For this review, take the finished solid that the model builds, in its own axes (mm). Face numbers are marked on the shaded views. A direction names the side the tool comes from. Coordinates: 2 decimals unless noted, no trailing zeros. Order: outer loops, then holes, each group sorted by start corner. A loop starts at its lowest first (then second) coordinate and runs counter-clockwise, first axis right, second up. Notation, with made-up numbers: M -8,-35 L 42,-35 A13 ccw 42,-20 Z; hole C 22.5,-36 d3. An arc over 180 degrees is marked long. Use CSV: the item, a comma, the result in double quotes.
```python
from build123d import *

# Parameters (mm, degrees)
F1_DEPTH = 50.8
F2_R     = 5.08
F3_R     = 5.08
F4_R     = 3.175
F5_DEPTH = 25.4


with BuildPart() as f1:
    # F0 (on Front) → F1 (new body)
    with BuildSketch(Plane.XZ):
        with BuildLine():
            Line((-25, -25), (-25, 0))
            Line((-25, 0), (-20, 0))
            ThreePointArc((-20, 0), (0, 20), (20, 0))
            Line((20, 0), (25, 0))
            Line((25, 0), (25, -25))
            Line((25, -25), (46.55, -25))
            Line((46.55, -25), (46.55, -22))
            Line((46.55, -22), (27.5, -22))
            Line((27.5, -22), (27.5, 0))
            Line((27.5, 0), (27.5, 25))
            Line((27.5, 25), (-27.5, 25))
            Line((-27.5, 25), (-27.5, 0))
            Line((-27.5, 0), (-27.5, -22))
            Line((-27.5, -22), (-46.55, -22))
            Line((-46.55, -22), (-46.55, -25))
            Line((-46.55, -25), (-25, -25))
        make_face()
    extrude(amount=F1_DEPTH)

    # F2
    f2_edges = [f1.edges().sort_by_distance(p)[0] for p in [
        (-27.5, -25.4, 25),
        (27.5, -25.4, 25),
    ]]
    fillet(f2_edges, radius=F2_R)

    # F3
    f3_edges = [f1.edges().sort_by_distance(p)[0] for p in [
        (-27.5, -25.4, -22),
        (27.5, -25.4, -22),
    ]]
    fillet(f3_edges, radius=F3_R)

    # F4 (on face) → F5 (cut)
    with BuildSketch(Plane.XY.offset(-22)):
        with Locations((-37.7, -25.4)):
            Circle(F4_R)
        with Locations((37.7, -25.4)):
            Circle(F4_R)
    extrude(amount=-F5_DEPTH, mode=Mode.SUBTRACT)


solid = f1.part
```
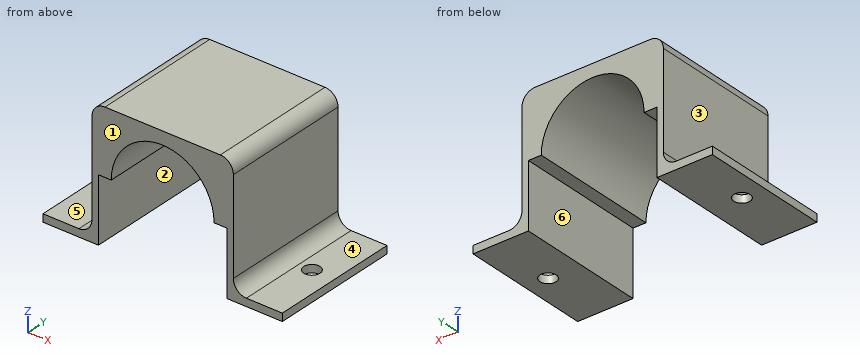
Item 1: Add section C-C on z = -2. State the section outline as (x, y) points.
Solutions:
outline,"M -27.5,-50.8 L -25,-50.8 L -25,0 L -27.5,0 Z; M 25,-50.8 L 27.5,-50.8 L 27.5,0 L 25,0 Z"
Item 2: To check wall thickness, follow line 1 along Y through (x, z) = (37.7, -23.85) (3 decimals); line 2 along Z through (x, y) = (33.5, -5); line 3 along X through (y, z) = (-45, -13.5). State the ranges of each line that lie inside material, in increasing order. Write a range as [from, to].
Solutions:
line 1,"[-50.8, -28.575], [-22.225, 0]"
line 2,"[-25, -22]"
line 3,"[-27.5, -25], [25, 27.5]"
Item 3: Draft analysis for pull direction X (two halves, no side actions). For the marked faces 1, 2 and 3, state which applies: released by +X, released by -X, zero draft, split by the parting line, or undercut.
Solutions:
face 1,"zero draft"
face 2,"undercut"
face 3,"released by -X"
Item 4: For the marked faces 4, 5 and 6, list the 3-axis set-ups (+Z, -Z, +X, -X, +Y, -Y) from which the entire face can be reached by the end or side of a thin tool; tool diameter is ignored.
Solutions:
face 4,"+Z, +X, +Y, -Y"
face 5,"+Z, -X, +Y, -Y"
face 6,"-Z, +Y, -Y"
Item 5: Add section D-D on y = -33. State the section outline as (x, z) points.
Solutions:
outline,"M -46.55,-25 L -25,-25 L -25,0 L -20,0 A20 cw 20,0 L 25,0 L 25,-25 L 46.55,-25 L 46.55,-22 L 32.58,-22 A5.08 cw 27.5,-16.92 L 27.5,19.92 A5.08 ccw 22.42,25 L -22.42,25 A5.08 ccw -27.5,19.92 L -27.5,-16.92 A5.08 cw -32.58,-22 L -46.55,-22 Z"
Item 6: Add section A-A on y = -25.4. State the section outline as (x, z) points (3 decimals), and give its area (3 significant figures).
Solutions:
outline,"M -46.55,-25 L -40.875,-25 L -40.875,-22 L -46.55,-22 Z; M -34.525,-25 L -25,-25 L -25,0 L -20,0 A20 cw 20,0 L 25,0 L 25,-25 L 34.525,-25 L 34.525,-22 L 32.58,-22 A5.08 cw 27.5,-16.92 L 27.5,19.92 A5.08 ccw 22.42,25 L -22.42,25 A5.08 ccw -27.5,19.92 L -27.5,-16.92 A5.08 cw -32.58,-22 L -34.525,-22 Z; M 40.875,-25 L 46.55,-25 L 46.55,-22 L 40.875,-22 Z"
area,"948 mm^2"
Item 7: Add section B-B on x = 37.7. State the section outline as (y, z) points (3 decimals).
Solutions:
outline,"M -50.8,-25 L -28.575,-25 L -28.575,-22 L -50.8,-22 Z; M -22.225,-25 L 0,-25 L 0,-22 L -22.225,-22 Z"
Item 8: Clearance check with flat-ended pins moving along their axes: pin 1 Ø5.5 at (x, y) = (-21.5, -19.5) entering from -Z; pin 2 Ø7.5 at (x, y) = (37.7, -25.4) entering from +Z; pin 3 Ø11 at (y, z) = (-34, 6.5) entering from +X. State where each tip first meets the part, or that it passes through.
Solutions:
pin 1,"z = 0"
pin 2,"z = -22"
pin 3,"x = 27.5"
